from build123d import *

# Parameters (mm, degrees)
SKETCH_1_W          = 20
SKETCH_1_H          = 20
SKETCH_1_W_2        = 18
SKETCH_1_H_2        = 18
EXTRUDE_1_DEPTH     = 270
SKETCH_2_R          = 1.6
CUT_EXTRUDE_1_DEPTH = 271.924343683
CUT_EXTRUDE_2_REACH = 272.924
SKETCH_3_W          = 18
SKETCH_3_H          = 18
SKETCH_4_R          = 1.6
CUT_EXTRUDE_3_DEPTH = 271.924343683
SKETCH_5_R          = 1.6
CUT_EXTRUDE_4_DEPTH = 271.924343683


with BuildPart() as part:
    # 草图1 → 凸台-拉伸1 (new body)
    with BuildSketch(Plane.XY):
        Rectangle(SKETCH_1_W, SKETCH_1_H)
        Rectangle(SKETCH_1_W_2, SKETCH_1_H_2, mode=Mode.SUBTRACT)
    extrude(amount=EXTRUDE_1_DEPTH)

    # 草图2 → 切除-拉伸1 (cut, through all)
    with BuildSketch(Plane(origin=(0, 10, 0), x_dir=(1, 0, 0), z_dir=(0, 1, 0))):
        with Locations(Location((-4.5, -179.5, 0), (0, 0, 270))):
            Circle(SKETCH_2_R)
        with Locations(Location((4.5, -179.5, 0), (0, 0, 270))):
            Circle(SKETCH_2_R)
        with Locations(Location((4.5, -170.5, 0), (0, 0, 270))):
            Circle(SKETCH_2_R)
        with Locations(Location((-4.5, -170.5, 0), (0, 0, 270))):
            Circle(SKETCH_2_R)
        with Locations(Location((-4.5, -99.5, 0), (0, 0, 270))):
            Circle(SKETCH_2_R)
        with Locations(Location((4.5, -90.5, 0), (0, 0, 270))):
            Circle(SKETCH_2_R)
        with Locations(Location((4.5, -99.5, 0), (0, 0, 270))):
            Circle(SKETCH_2_R)
        with Locations(Location((-4.5, -90.5, 0), (0, 0, 270))):
            Circle(SKETCH_2_R)
    extrude(amount=-CUT_EXTRUDE_1_DEPTH, mode=Mode.SUBTRACT)

    # 草图3 → 切除-拉伸2 (cut, up to next)
    with BuildSketch(Plane.XZ.offset(10), mode=Mode.PRIVATE) as cut_extrude_2_sk1:
        with Locations((0, 175)):
            Rectangle(SKETCH_3_W, SKETCH_3_H)
    cut_extrude_2_tool1 = extrude(cut_extrude_2_sk1.sketch, amount=-CUT_EXTRUDE_2_REACH, mode=Mode.PRIVATE) & part.part
    # 草图3 → 切除-拉伸2 (cut, up to next)
    with BuildSketch(Plane.XZ.offset(10), mode=Mode.PRIVATE) as cut_extrude_2_sk2:
        with Locations((0, 95)):
            Rectangle(SKETCH_3_W, SKETCH_3_H)
    cut_extrude_2_tool2 = extrude(cut_extrude_2_sk2.sketch, amount=-CUT_EXTRUDE_2_REACH, mode=Mode.PRIVATE) & part.part
    add(cut_extrude_2_tool1.solids().sort_by_distance((0, -10, 175))[0], mode=Mode.SUBTRACT)
    add(cut_extrude_2_tool2.solids().sort_by_distance((0, -10, 95))[0], mode=Mode.SUBTRACT)

    # 草图4 → 切除-拉伸3 (cut, through all)
    with BuildSketch(Plane(origin=(0, 10, 0), x_dir=(1, 0, 0), z_dir=(0, 1, 0))):
        with Locations(Location((-4.5, -5.5, 0), (0, 0, 270))):
            Circle(SKETCH_4_R)
        with Locations(Location((4.5, -5.5, 0), (0, 0, 270))):
            Circle(SKETCH_4_R)
        with Locations(Location((-4.5, -264.5, 0), (0, 0, 270))):
            Circle(SKETCH_4_R)
        with Locations(Location((4.5, -264.5, 0), (0, 0, 90))):
            Circle(SKETCH_4_R)
    extrude(amount=-CUT_EXTRUDE_3_DEPTH, mode=Mode.SUBTRACT)

    # 草图5 → 切除-拉伸4 (cut, through all)
    with BuildSketch(Plane.XZ.offset(10)):
        with Locations(Location((0, 56, 0), (0, 0, 270))):
            Circle(SKETCH_5_R)
        with Locations(Location((0, 40, 0), (0, 0, 270))):
            Circle(SKETCH_5_R)
    cut_extrude_4 = extrude(amount=-CUT_EXTRUDE_4_DEPTH, mode=Mode.SUBTRACT)

    # 镜向1: 切除-拉伸4 across plane
    add(cut_extrude_4.mirror(Plane(origin=(0, 0, 135), x_dir=(1, 0, 0), z_dir=(0, 0, -1))), mode=Mode.SUBTRACT)


solid = part.part
Geometry: final body of the model. Coordinates: model frame, mm. A direction names the side the tool comes from. Give positions to 0.01 mm unless a question says otherwise; leave off trailing zeros. Order: outer loops, then holes, each group sorted by start corner. A loop starts at its lowest first (then second) coordinate and runs counter-clockwise, first axis right, second up. Notation, with made-up numbers: (65, 46) -> (110, 46) arc R25 cw to (110, 60) -> close; hole circle Ø2 at (26, 67.5). An arc over 180 degrees is marked (long way). Write each question's results on one line, items separated by ' | '.
1) Draft query along Y for faces 3 (the face through (0, -10, 133)), 4 (the face through (-0.8, -9.6, 270)), 5 (the face through (0, -9, 226)). Return one class per face: released by +Y, released by -Y, zero draft, split by the parting line, or undercut.
Geometry says:
face 3: released by -Y | face 4: zero draft | face 5: undercut
2) Cut plane A-A (y = -4.5). Output: boundary loops of the cut face in (x, z), and give its area (3 significant figures).
Geometry says:
outline: (-10, 0) -> (-9, 0) -> (-9, 270) -> (-10, 270) -> close; (9, 0) -> (10, 0) -> (10, 270) -> (9, 270) -> close | area: 540 mm²
3) Line query: line 1 along X through (y, z) = (9.4, 99.5); line 2 along Y through (x, z) = (-8, 82); line 3 along X through (y, z) = (9.6, 40). Output: solid intervals per line, ascending.
Geometry says:
line 1: x = -10 to -6.1, -2.9 to 2.9, 6.1 to 10 | line 2: y = -10 to -9, 9 to 10 | line 3: x = -10 to -1.6, 1.6 to 10
4) First-contact query: pin 1 Ø5 at (x, z) = (4.5, 99.5) entering from +Y; pin 2 Ø1.9 at (x, z) = (0, 230) entering from -Y; pin 3 Ø5 at (x, z) = (4.5, 90.5) entering from -Y. Flat tips, straight axial feed; report the tip coordinate or a pass-through.
Geometry says:
pin 1: stops at y = 10 | pin 2: passes through | pin 3: stops at y = 9
5) Cut plane B-B (z = 201). Output: boundary loops of the cut face in (x, y).
Geometry says:
outline: (-10, -10) -> (10, -10) -> (10, 10) -> (-10, 10) -> close; hole (-9, -9) -> (9, -9) -> (9, 9) -> (-9, 9) -> close
6) Set-up query: faces 1 (the face through (0, 9, 133)), 2 (the face through (-10, 0, 133)). Return all of +Z, -Z, +X, -X, +Y, -Y with unobstructed straight access to the full face (end or side cutting, diameter ignored); none if empty.
Geometry says:
face 1: +Z, -Z | face 2: +Z, -Z, -X, +Y, -Y
